Answer from the drawing. Dimensions are ordinates in mm from the lowest x, y and z of the part. A direction names the side the tool comes from. Give positions to 0.01 mm unless a question says otherwise; leave off trailing zeros. Write each loop counter-clockwise with the first axis right and the second up, starting at its lowest first coordinate (ties: lowest second). Pieces come first, ordered by that corner, then holes. Notation, with made-up numbers: (0.25, 56.25) -> (39.25, 56.25) arc R6 cw to (39.25, 67.25) -> close; hole circle Ø3 at (-2.5, -30.5). An arc over 180 degrees is marked (long way). Use a Markdown table: item, result. Add a question column.
Q1. Section C-C, the plane z = 9 is taken. Give the vertices of the cut face in (x, y), plus the area to 3 significant figures.
Q2. Consider line 1 (Y direction, x = 4, z = 9.15); line 2 (Z direction, x = 4, y = 9); line 3 (X direction, y = 4.5, z = 9). Determine where each line is inside the solid, lowest interval first.
Q3. Section A-A, the plane y = 2.75 is taken. Give the vertices of the cut face in (x, z).
Q4. Section B-B, the plane x = 4 is taken. Give the vertices of the cut face in (y, z).
Q5. Each of these flat-tipped pins is pushed along its axis until it touches: pin 1 Ø1.5 at (x, y) = (3.5, 8) entering from +Z; pin 2 Ø1.2 at (y, z) = (8.5, 2) entering from +X. Where does it stop, or does it pass through?
Q6. For the marked faces 4, 5 and 6, determine the directions among +Z, -Z, +X, -X, +Y, -Y from which every point of the face is accessible in a straight line to the end or side of a thin tool.
Q7. Section D-D, the plane y = 5.25 is taken. Give the vertices of the cut face in (x, z).
Q8. For a pull along Z with two mould halves and no side action, classify the marked faces 1, 2 and 3 as pulls with the +Z half, pulls with the -Z half, needs draft (parallel to the pull), parting line crosses it, or undercut.
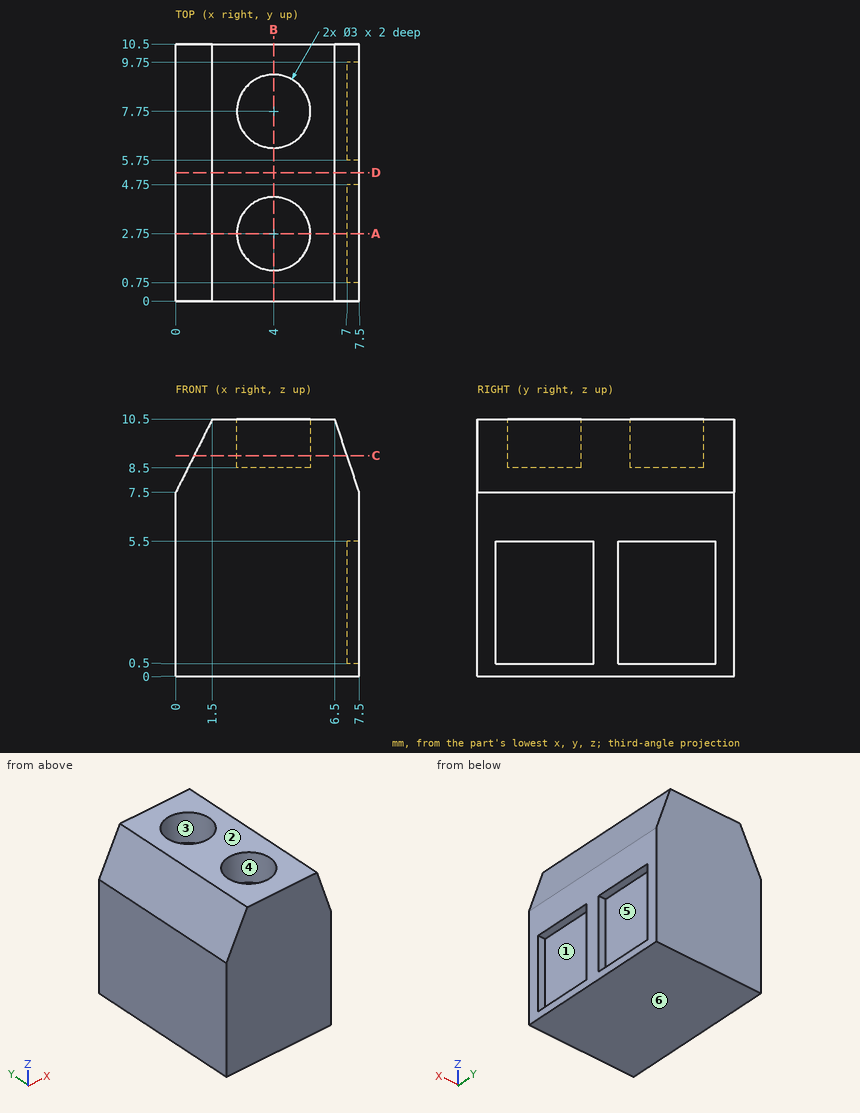
Result set:
| question | item | result |
|---|---|---|
| 1 | outline | (0.75, 0) -> (7, 0) -> (7, 10.5) -> (0.75, 10.5) -> close; hole circle Ø3 at (4, 2.75); hole circle Ø3 at (4, 7.75) |
| 1 | area | 51.5 mm2 |
| 2 | line 1 | y = 0 to 1.25, 4.25 to 6.25, 9.25 to 10.5 |
| 2 | line 2 | z = 0 to 8.5 |
| 2 | line 3 | x = 0.75 to 7 |
| 3 | outline | (0, 0) -> (7.5, 0) -> (7.5, 0.5) -> (7, 0.5) -> (7, 5.5) -> (7.5, 5.5) -> (7.5, 7.5) -> (6.5, 10.5) -> (5.5, 10.5) -> (5.5, 8.5) -> (2.5, 8.5) -> (2.5, 10.5) -> (1.5, 10.5) -> (0, 7.5) -> close |
| 4 | outline | (0, 0) -> (10.5, 0) -> (10.5, 10.5) -> (9.25, 10.5) -> (9.25, 8.5) -> (6.25, 8.5) -> (6.25, 10.5) -> (4.25, 10.5) -> (4.25, 8.5) -> (1.25, 8.5) -> (1.25, 10.5) -> (0, 10.5) -> close |
| 5 | pin 1 | stops at z = 8.5 |
| 5 | pin 2 | stops at x = 7 |
| 6 | face 4 | +Z |
| 6 | face 5 | +X |
| 6 | face 6 | -Z, +X, -X, +Y, -Y |
| 7 | outline | (0, 0) -> (7.5, 0) -> (7.5, 7.5) -> (6.5, 10.5) -> (1.5, 10.5) -> (0, 7.5) -> close |
| 8 | face 1 | undercut |
| 8 | face 2 | pulls with the +Z half |
| 8 | face 3 | needs draft |
